Part model, mm, in its own coordinate system. A direction names the side the tool comes from. Round coordinates to 2 decimals unless told otherwise and drop trailing zeros. Write each loop counter-clockwise with the first axis right and the second up, starting at its lowest first coordinate (ties: lowest second). Pieces come first, ordered by that corner, then holes. Notation, with made-up numbers: (23, 76) -> (38, 76) arc R27 ccw to (38, 107) -> close; hole circle Ø1 at (-31, 67.5). An arc over 180 degrees is marked (long way). Return JSON: item names as keys, results as strings. Group by question number.
Autodesk Inventor part; units mm, degrees
ref_plane "YZ Plane" through (0, 0, 0) normal (1, 0, 0) x (0, 1, 0)
ref_plane "XZ Plane" through (0, 0, 0) normal (0, 1, 0) x (-1, 0, 0)
ref_plane "XY Plane" through (0, 0, 0) normal (0, 0, 1) x (1, 0, 0)
sketch "Sketch1" plane through (0, 0, 0) normal (1, 0, 0) x (0, 1, 0)
  point P0 (0, 0)
sketch "Sketch2" plane through (0, 0, 0) normal (0, 0, 1) x (1, 0, 0)
  line L0 (0, 0) -> (20, 0)
  line L1 (20, 0) -> (20, 3)
  line L2 (0, 0) -> (0, 3)
  line L3 (0, 3) -> (6.0777, 37.4683)
  line L4 (0, 3) -> (35, 3) construction
  line L5 (6.0777, 37.4683) -> (9.0321, 36.9473)
  line L6 (9.0321, 36.9473) -> (3.0463, 3)
  line L7 (3.0463, 3) -> (20, 3)
  dimension "d0" = 20
  dimension "d1" = 3
  dimension "d2" = 3
  dimension "d4" = 35
  dimension "d5" = 80
  dimension "d6" = 3
extrude "Extrusion1" add sketch "Sketch2" along normal blind 26 and the other way blind 26
ref_plane "Work Plane1" through (7.5549, 37.2078, 26) normal (0.9848, -0.1736, 0) x (0, 0, -1)
ref_plane "Work Plane2" through (0, 0, 0) normal (0, 0, 1) x (1, 0, 0)
sketch "Sketch3" plane through (9.0321, 36.9473, 26) normal (0.9848, -0.1736, 0) x (0, 0, -1)
  point P0 (26, -37.9544)
sketch "Sketch4" plane through (9.0321, 36.9473, 26) normal (0.9848, -0.1736, 0) x (0, 0, -1)
  circle A0 centre (3.5, -8.527) radius 1.5
  circle A1 centre (48.5, -8.527) radius 1.5
  point P0 (26, -37.9544)
  dimension "d11" = 3
  dimension "d12" = 3
extrude "Extrusion2" cut sketch "Sketch4" against normal blind 3 contours A0
sketch "Sketch5" plane through (9.0321, 36.9473, 26) normal (0.9848, -0.1736, 0) x (0, 0, -1)
  circle A0 centre (48.5, -8.527) radius 1.5
  point P0 (26, -37.9544)
  dimension "d15" = 3
extrude "Extrusion3" cut sketch "Sketch5" against normal blind 3
sketch "Sketch6" plane through (3.0463, 3, 26) normal (0, 1, 0) x (1, 0, 0)
  point P0 (-3.0463, 26)
sketch "Sketch7" plane through (0, 0, 26) normal (0, -1, 0) x (1, 0, 0)
  line L0 (6.0777, -52) -> (6.0777, 0)
  line L1 (5, -3) -> (17, -3)
  line L2 (17, -7) -> (5, -7)
  arc A0 (17, -7) -> (17, -3) centre (17, -5) ccw
  line L3 (5, -3) -> (5, -7)
  ellipse E0 centre (4.597, -3.5) end of major axis (4.597, -2) minor radius 0.2605
  line L4 (20, -52) -> (20, 0)
  line L5 (5, -49) -> (17, -49)
  line L6 (17, -45) -> (5, -45)
  arc A1 (17, -49) -> (17, -45) centre (17, -47) ccw
  line L7 (5, -49) -> (5, -45)
  point P0 (0, -26)
  dimension "d19" = 12
extrude "Extrusion4" cut sketch "Sketch7" against normal blind 3 contours L5 L7 L6 L0 | L2 L3 L1 L0 | L0 L1 A0 L2 | L0 L6 A1 L5
Item 1: Cut at C-C (z = 13). Write the cut outline in (x, y), then the cut area to 3 significant figures.
Item 2: Cut at B-B (z = -20). Write the cut outline in (x, y).
Item 3: Cut at A-A (x = 13.5). Write the cut outline in (y, z), then the cut area to 3 significant figures.
Item 4: Flat gauge pins, fed straight in: P1, Ø1.5, axis at y = 4.5, z = -16, coming from the -X side; P2, Ø2, axis at x = 8, z = 9.5, coming from the +Y side; P3, Ø2, axis at x = 14, z = -11, coming from the +Y side. Where does each tip first touch, or does it go through?
Item 5: Cut at D-D (y = 28). State how many separate pieces and enclosed holes the cut face has, then the cut area to 3 significant figures.
Item 6: Two-plate mould, pull along X, no slides. Class faces 1 (the face through (11, 3, 0)), 2 (the face through (20, 1, 0)), 3 (the face through (11, 1, 23)), 4 (the face through (2.996, 19.993, -0.364)): released by +X, released by -X, zero draft, split by the parting line, or undercut.
Item 7: Which spindle directions (+Z, -Z, +X, -X, +Y, -Y) get a long thin tool onto all of the face, cutting with end or side? Do faces 5 (the face through (10, 0, 0)), 6 (the face through (19, 1, -21)), 7 (the face through (11, 1, -19)), 8 (the face through (6.08, 20.21, -0.36)). Say none if no direction does.
Item 8: Wall check: L1, parallel to Y at x = 18.5, z = 12; L2, parallel to X at y = 5, z = 9.5; L3, parallel to X at y = 16, z = 22.5. Give the ranges that are in metal, low to high.
Checks:
{
 "1": {"outline": "(0, 0) -> (20, 0) -> (20, 3) -> (3.05, 3) -> (9.03, 36.95) -> (6.08, 37.47) -> (0, 3) -> close", "area": "164 mm2"},
 "2": {"outline": "(0, 0) -> (5, 0) -> (5, 3) -> (3.05, 3) -> (9.03, 36.95) -> (6.08, 37.47) -> (0, 3) -> close; (18.73, 0) -> (20, 0) -> (20, 3) -> (18.73, 3) -> close"},
 "3": {"outline": "(0, -26) -> (3, -26) -> (3, -23) -> (0, -23) -> close; (0, -19) -> (3, -19) -> (3, 19) -> (0, 19) -> close; (0, 23) -> (3, 23) -> (3, 26) -> (0, 26) -> close", "area": "132 mm2"},
 "4": {"P1": "stops at x = 0.13", "P2": "stops at y = 37.31", "P3": "stops at y = 3"},
 "5": {"separate pieces": "3", "enclosed holes": "0", "area": "143 mm2"},
 "6": {"face 1": "zero draft", "face 2": "released by +X", "face 3": "undercut", "face 4": "released by -X"},
 "7": {"face 5": "+Z, -Z, +X, -X, -Y", "face 6": "+Y, -Y", "face 7": "-Y", "face 8": "+Z, -Z, +X"},
 "8": {"L1": "y = 0 to 3", "L2": "x = 0.35 to 3.4", "L3": "x = 2.29 to 5.34"}
}
